Autodesk Inventor part; units mm, degrees
ref_plane "YZ Plane" through (0, 0, 0) normal (1, 0, 0) x (0, 1, 0)
ref_plane "XZ Plane" through (0, 0, 0) normal (0, 1, 0) x (-1, 0, 0)
ref_plane "XY Plane" through (0, 0, 0) normal (0, 0, 1) x (1, 0, 0)
sketch "Sketch1" plane through (0, 0, 0) normal (0, 1, 0) x (-1, 0, 0)
  line L0 (0, 0) -> (14.732, 0)
  line L1 (14.732, 0) -> (14.732, -12.7)
  line L2 (14.732, -12.7) -> (0, -12.7)
  line L3 (0, -12.7) -> (0, 0)
  dimension "d0" = 12.7
  dimension "d1" = 14.732
extrude "Extrusion1" add sketch "Sketch1" along normal blind 26.67
sketch "Sketch2" plane through (0, 0, -12.7) normal (0, 0, -1) x (-1, 0, 0)
  line L0 (0, 0) -> (14.732, 0)
  line L1 (14.732, 0) -> (14.732, 2.54)
  line L2 (14.732, 0) -> (14.732, 26.67)
  line L3 (14.732, 2.54) -> (14.732, 6.604)
  line L4 (14.732, 6.604) -> (0, 6.604)
  line L5 (0, 0) -> (0, 26.67)
  line L6 (14.732, 2.54) -> (0, 2.54)
  line L7 (0, 2.54) -> (0, 6.604)
  line L8 (0, 6.604) -> (14.732, 6.604)
  line L9 (14.732, 6.604) -> (14.732, 2.54)
  dimension "d4" = 2.54
  dimension "d5" = 4.064
extrude "Extrusion2" cut sketch "Sketch2" against normal blind 10.414 contours L5 L4 L2 L6
sketch "Sketch3" plane through (0, 0, 0) normal (1, 0, 0) x (0, 0, -1)
  line L0 (0, 26.67) -> (12.7, 26.67)
  line L1 (0, 26.67) -> (6.35, 26.67)
  line L2 (6.35, 26.67) -> (6.35, 20.32)
  line L3 (6.35, 20.32) -> (3.175, 20.32)
  line L4 (3.175, 20.32) -> (3.175, 17.78)
  line L5 (3.175, 20.32) -> (9.525, 20.32)
  line L6 (9.525, 20.32) -> (9.525, 17.78)
  line L7 (9.525, 17.78) -> (3.175, 17.78)
  line L8 (3.175, 17.78) -> (3.175, 20.32)
  point P0 (0, 0)
  dimension "d8" = 6.35
  dimension "d9" = 6.35
  dimension "d10" = 3.175
  dimension "d11" = 2.54
  dimension "d12" = 6.35
extrude "Extrusion3" cut sketch "Sketch3" against normal blind 15.1765
properties part number "drone_battery_holder"
The listing builds one solid part. Answer for the finished solid, in the listing's coordinates (mm). A direction names the side the tool comes from. Give positions to 0.01 mm unless a question says otherwise; leave off trailing zeros. Order: outer loops, then holes, each group sorted by start corner. A loop starts at its lowest first (then second) coordinate and runs counter-clockwise, first axis right, second up. Notation, with made-up numbers: (21, 32) -> (29, 32) arc R19 cw to (29, 60) -> close; hole circle Ø2 at (13.25, -16.75). An arc over 180 degrees is marked (long way). One line per item, written item: value.
1) Determine the mould class of faces 4 (the flat face through (-7, 19, -9.525)), 5 (the flat face through (-7, 26.67, -6)), 6 (the flat face through (-7, 0, -6)) for opening direction Y: pulls with the +Y half, pulls with the -Y half, needs draft (parallel to the pull), parting line crosses it, or undercut.
Reported:
face 4: undercut
face 5: pulls with the +Y half
face 6: pulls with the -Y half
2) Find section A-A, the plane z = -5. Determine the outline of the cut face in (x, y).
Reported:
outline: (-14.73, 0) -> (0, 0) -> (0, 2.54) -> (-14.73, 2.54) -> close; (-14.73, 6.6) -> (0, 6.6) -> (0, 17.78) -> (-14.73, 17.78) -> close; (-14.73, 20.32) -> (0, 20.32) -> (0, 26.67) -> (-14.73, 26.67) -> close
3) A flat-ended cylindrical pin translates along its axis: P1, Ø1, axis at y = 7, z = -3, coming from the +X side. Find the tip coordinate at first contact, or state that the pin passes through.
Reported:
P1: stops at x = 0
4) Find section C-C, the plane z = -11.5. Determine the outline of the cut face in (x, y), plus the area to 3 significant figures.
Reported:
outline: (-14.73, 0) -> (0, 0) -> (0, 2.54) -> (-14.73, 2.54) -> close; (-14.73, 6.6) -> (0, 6.6) -> (0, 26.67) -> (-14.73, 26.67) -> close
area: 333 mm^2
5) Find the intervals of material crossed by line 1 (Y direction, x = -4.25, z = -8.75); line 2 (Y direction, x = -5, z = -2.5); line 3 (Z direction, x = -4.5, y = 6.5), in increasing order.
Reported:
line 1: y = 0 to 2.54, 6.6 to 17.78, 20.32 to 26.67
line 2: y = 0 to 2.54, 6.6 to 26.67
line 3: z = -2.29 to 0
6) Find section B-B, the plane x = -12.75. Determine the outline of the cut face in (y, z) (3 decimals).
Reported:
outline: (0, -12.7) -> (2.54, -12.7) -> (2.54, -2.286) -> (6.604, -2.286) -> (6.604, -12.7) -> (26.67, -12.7) -> (26.67, 0) -> (0, 0) -> close; hole (17.78, -9.525) -> (20.32, -9.525) -> (20.32, -3.175) -> (17.78, -3.175) -> close
7) A tool of negligible diameter and unlimited length cuts with its end or side. For faces 1 (the flat face through (-7, 20.32, -6)), 2 (the flat face through (-7, 5, -2.286)), 3 (the flat face through (-7, 13, 0)), from which of +Z, -Z, +X, -X, +Y, -Y can it reach the whole face along a straight path? Write none if from no direction.
Reported:
face 1: +X, -X
face 2: -Z, +X, -X
face 3: +Z, +X, -X, +Y, -Y
